```python
from build123d import *

# Parameters (mm, degrees)
SKETCH1_W           = 60
SKETCH1_H           = 115
BOSS_EXTRUDE1_DEPTH = 15
SKETCH2_R           = 7.5
SKETCH2_R_2         = 5
CUT_EXTRUDE1_DEPTH  = 10
SKETCH3_R           = 5
CUT_EXTRUDE2_DEPTH  = 14.5
SKETCH4_R           = 4.75
BOSS_EXTRUDE2_DEPTH = 30
FILLET1_R           = 1
FILLET2_R           = 10
SKETCH5_R           = 4.826
SKETCH5_R_2         = 2.413
BOSS_EXTRUDE3_DEPTH = 5


with BuildPart() as part:
    # Sketch1 → Boss-Extrude1 (new body)
    with BuildSketch(Plane(origin=(0, 0, 0), x_dir=(1, 0, 0), z_dir=(0, 1, 0))):
        with Locations((30, 57.5)):
            Rectangle(SKETCH1_W, SKETCH1_H)
    extrude(amount=BOSS_EXTRUDE1_DEPTH)

    # Sketch2 → Cut-Extrude1 (cut)
    with BuildSketch(Plane(origin=(0, 15, 0), x_dir=(1, 0, 0), z_dir=(0, 1, 0))):
        with Locations((30, 93.55)):
            Circle(SKETCH2_R)
        with Locations((30, 11.45)):
            Circle(SKETCH2_R_2)
    extrude(amount=-CUT_EXTRUDE1_DEPTH, mode=Mode.SUBTRACT)

    # Sketch3 → Cut-Extrude2 (cut)
    with BuildSketch(Plane(origin=(0, 0, 0), x_dir=(-1, 0, 0), z_dir=(0, -1, 0))):
        with Locations((-30, 57.5)):
            Circle(SKETCH3_R)
    extrude(amount=-CUT_EXTRUDE2_DEPTH, mode=Mode.SUBTRACT)

    # Sketch4 → Boss-Extrude2 (add)
    with BuildSketch(Plane(origin=(0, 5, 0), x_dir=(1, 0, 0), z_dir=(0, 1, 0))):
        with Locations((30, 11.45)):
            Circle(SKETCH4_R)
    extrude(amount=BOSS_EXTRUDE2_DEPTH)

    # Fillet1
    fillet1_edges = [part.edges().sort_by_distance(p)[0] for p in [
        (25.25, 35, -11.45),
    ]]
    fillet(fillet1_edges, radius=FILLET1_R)

    # Fillet2
    fillet2_edges = [part.edges().sort_by_distance(p)[0] for p in [
        (0, 7.5, -115),
        (60, 7.5, -115),
        (60, 7.5, 0),
        (0, 7.5, 0),
    ]]
    fillet(fillet2_edges, radius=FILLET2_R)

    # Sketch5 → Boss-Extrude3 (add)
    with BuildSketch(Plane(origin=(0, 15, 0), x_dir=(1, 0, 0), z_dir=(0, 1, 0))):
        with Locations((50, 62.5)):
            Circle(SKETCH5_R)
        with Locations((50, 62.5)):
            Circle(SKETCH5_R_2, mode=Mode.SUBTRACT)
        with Locations((50, 32.5)):
            Circle(SKETCH5_R)
        with Locations((50, 32.5)):
            Circle(SKETCH5_R_2, mode=Mode.SUBTRACT)
        with Locations((10, 32.5)):
            Circle(SKETCH5_R)
        with Locations((10, 32.5)):
            Circle(SKETCH5_R_2, mode=Mode.SUBTRACT)
        with Locations((10, 62.5)):
            Circle(SKETCH5_R)
        with Locations((10, 62.5)):
            Circle(SKETCH5_R_2, mode=Mode.SUBTRACT)
    extrude(amount=BOSS_EXTRUDE3_DEPTH)


solid = part.part
```
The model under review builds one solid part; all positions refer to its coordinate system, in mm. A direction names the side the tool comes from. Round coordinates to 2 decimals unless told otherwise and drop trailing zeros. Order: outer loops, then holes, each group sorted by start corner. A loop starts at its lowest first (then second) coordinate and runs counter-clockwise, first axis right, second up.
(1) Take a section at B-B, the plane y = 2. State the section outline as (x, z) points, plus the area to 3 significant figures.
Working result:
outline: (0, -105) arc R10 ccw to (10, -115) - (50, -115) arc R10 ccw to (60, -105) - (60, -10) arc R10 ccw to (50, 0) - (10, 0) arc R10 ccw to (0, -10) - close; hole circle Ø10 at (30, -57.5)
area: 6,740 mm2
(2) Take a section at A-A, the plane y = 18. Count the separate pieces of the cut face and the enclosed holes in it, plus the area to 3 significant figures.
Working result:
separate pieces: 5
enclosed holes: 4
area: 290 mm2
(3) Tool access review of faces 1 (the face through (11, 20, -65)), 2 (the face through (10, 15, -63)): name each direction out of +Z, -Z, +X, -X, +Y, -Y from which nothing blocks a thin tool from reaching the whole face with its end or side.
Working result:
face 1: +Z, -Z, +X, -X, +Y
face 2: +Y
(4) Take a section at D-D, the plane x = 39. State the section outline as (y, z) points, plus the area to 4 significant figures.
Working result:
outline: (0, -115) - (15, -115) - (15, 0) - (0, 0) - close
area: 1,725 mm2
(5) Mouldability with a two-part tool opening along Z and no side actions: class faces 3 (the face through (30, 7, -115)), 4 (the face through (11, 20, -35)), 5 (the face through (6.17, 17.465, -29.563)) as released by +Z, released by -Z, zero draft, split by the parting line, or undercut.
Working result:
face 3: released by -Z
face 4: zero draft
face 5: undercut
(6) Wall thickness on L1, parallel to Z at x = 10, y = 18.85; L2, parallel to X at y = 18.8, z = -32.5; L3, parallel to Z at x = 30, y = 12: over which ranges is each line inside the solid? List them lowest first.
Working result:
L1: z = -67.33 to -64.91, -60.09 to -57.67, -37.33 to -34.91, -30.09 to -27.67
L2: x = 5.17 to 7.59, 12.41 to 14.83, 45.17 to 47.59, 52.41 to 54.83
L3: z = -115 to -101.05, -86.05 to -62.5, -52.5 to -16.45, -16.2 to -6.7, -6.45 to 0
(7) For P1, Ø6, axis at x = 8, z = -77, coming from the +Y side; P2, Ø5.5, axis at x = 49.5, z = -63, coming from the +Y side; P3, Ø8, axis at x = 37.5, y = 21, coming from the +Z side, all flat-tipped, find the tip position at first contact; note any pin that passes through.
Working result:
P1: stops at y = 15
P2: stops at y = 20
P3: stops at z = -8.24
(8) Take a section at C-C, the plane z = -11.45. State the section outline as (x, y) points.
Working result:
outline: (0, 0) - (60, 0) - (60, 15) - (35, 15) - (35, 5) - (34.75, 5) - (34.75, 34) arc R1 ccw to (33.75, 35) - (26.25, 35) arc R1 ccw to (25.25, 34) - (25.25, 5) - (25, 5) - (25, 15) - (0, 15) - close
